Design review of the part built by this model. Coordinates are the model's own, in mm. A direction names the side the tool comes from. Round coordinates to 2 decimals unless told otherwise and drop trailing zeros. Order: outer loops, then holes, each group sorted by start corner. A loop starts at its lowest first (then second) coordinate and runs counter-clockwise, first axis right, second up.
from build123d import *

# Parameters (mm, degrees)
SKETCH_1_W               = 45
SKETCH_1_H               = 80
SKETCH_1_R               = 1.6
EXTRUDE_471_DEPTH        = 20
SKETCH_2_R               = 2.6
CUT_EXTRUDE_665_DEPTH    = 46
SKETCH_3_R               = 5.1
CUT_EXTRUDE_863_DEPTH    = 46
SKETCH_5_W               = 30
SKETCH_5_H               = 20
CUT_EXTRUDE_1108_DEPTH   = 5.5
MIRROR_2_COPY_1_SKETCH_W = 30
MIRROR_2_COPY_1_SKETCH_H = 20
MIRROR_2_COPY_1_DEPTH    = 5.5
FILLET_2_R               = 2
FILLET_5_R               = 5


with BuildPart() as part:
    # 草图1 → Extrude 471 (new body)
    with BuildSketch(Plane(origin=(0, 0, 0), x_dir=(1, 0, 0), z_dir=(0, 1, 0))):
        Rectangle(SKETCH_1_W, SKETCH_1_H)
        with Locations((8, 15)):
            Circle(SKETCH_1_R, mode=Mode.SUBTRACT)
        with Locations((-8, 15)):
            Circle(SKETCH_1_R, mode=Mode.SUBTRACT)
        with Locations((-8, -15)):
            Circle(SKETCH_1_R, mode=Mode.SUBTRACT)
        with Locations((8, -15)):
            Circle(SKETCH_1_R, mode=Mode.SUBTRACT)
    extrude(amount=EXTRUDE_471_DEPTH)

    # 草图2 → Cut-Extrude 665 (cut, through all)
    with BuildSketch(Plane.ZY.offset(22.5)):
        with Locations((0, 10)):
            Circle(SKETCH_2_R)
    extrude(amount=-CUT_EXTRUDE_665_DEPTH, mode=Mode.SUBTRACT)

    # 草图3 → Cut-Extrude 863 (cut, through all)
    with BuildSketch(Plane.ZY.offset(22.5)):
        with Locations((22.5, 10)):
            Circle(SKETCH_3_R)
        with Locations((-22.5, 10)):
            Circle(SKETCH_3_R)
    extrude(amount=-CUT_EXTRUDE_863_DEPTH, mode=Mode.SUBTRACT)

    # 草图5 → Cut-Extrude 1108 (cut)
    with BuildSketch(Plane.ZY.offset(22.5)):
        with Locations((25, 10)):
            Rectangle(SKETCH_5_W, SKETCH_5_H)
    cut_extrude_1108 = extrude(amount=-CUT_EXTRUDE_1108_DEPTH, mode=Mode.SUBTRACT)

    # 镜向1: Cut-Extrude 1108 across plane
    add(cut_extrude_1108.mirror(Plane(origin=(0, 0, 0), x_dir=(0, 0, 1), z_dir=(1, 0, 0))), mode=Mode.SUBTRACT)

    # 镜向2: Cut-Extrude 1108 across plane
    add(cut_extrude_1108.mirror(Plane.XY), mode=Mode.SUBTRACT)

    # 镜向2 copy 1 sketch → 镜向2 copy 1 (cut)
    with BuildSketch(Plane(origin=(22.5, 0, 0), x_dir=(0, 0, -1), z_dir=(1, 0, 0))):
        with Locations((25, 10)):
            Rectangle(MIRROR_2_COPY_1_SKETCH_W, MIRROR_2_COPY_1_SKETCH_H)
    extrude(amount=-MIRROR_2_COPY_1_DEPTH, mode=Mode.SUBTRACT)

    # 圆角2
    fillet_2_edges = [part.edges().sort_by_distance(p)[0] for p in [
        (-22.5, 10, 10),
        (-17, 10, 10),
        (17, 10, 10),
        (22.5, 10, 10),
        (22.5, 10, -10),
        (17, 10, -10),
        (-17, 10, -10),
        (-22.5, 10, -10),
    ]]
    fillet(fillet_2_edges, radius=FILLET_2_R)

    # 圆角5
    fillet_5_edges = [part.edges().sort_by_distance(p)[0] for p in [
        (-17, 10, 40),
        (17, 10, 40),
        (17, 10, -40),
        (-17, 10, -40),
    ]]
    fillet(fillet_5_edges, radius=FILLET_5_R)


solid = part.part
1) Take a section at A-A on z = -22.5. Give the boundary of the cut face in (x, y), plus the area to 3 significant figures.
Results:
outline: (-17, 0) - (17, 0) - (17, 4.9) - (-17, 4.9) - close; (-17, 15.1) - (17, 15.1) - (17, 20) - (-17, 20) - close
area: 333 mm2
2) To check wall thickness, follow line 1 along X through (y, z) = (6, 15); line 2 along Y through (x, z) = (10, -22.5); line 3 along Z through (x, y) = (-2, 7.25). State the ranges of each line that lie inside material, in increasing order.
Results:
line 1: x = -17 to -9.6, -6.4 to 6.4, 9.6 to 17
line 2: y = 0 to 4.9, 15.1 to 20
line 3: z = -40 to -26.8, -18.2 to 18.2, 26.8 to 40
3) The part is to be moulded in two halves that separate along Z. For faces 1 (the face through (15, 10, 39)), 2 (the face through (-9.18, 9.86, 13.92)), 3 (the face through (17, 10, 28)), say which applies: released by +Z, released by -Z, zero draft, split by the parting line, or undercut.
Results:
face 1: released by +Z
face 2: undercut
face 3: zero draft
4) Take a section at C-C on y = 18.25. Give the boundary of the cut face in (x, z).
Results:
outline: (-22.5, -8) arc R2 ccw to (-20.5, -10) - (-19, -10) arc R2 cw to (-17, -12) - (-17, -35) arc R5 ccw to (-12, -40) - (12, -40) arc R5 ccw to (17, -35) - (17, -12) arc R2 cw to (19, -10) - (20.5, -10) arc R2 ccw to (22.5, -8) - (22.5, 8) arc R2 ccw to (20.5, 10) - (19, 10) arc R2 cw to (17, 12) - (17, 35) arc R5 ccw to (12, 40) - (-12, 40) arc R5 ccw to (-17, 35) - (-17, 12) arc R2 cw to (-19, 10) - (-20.5, 10) arc R2 ccw to (-22.5, 8) - close; hole circle Ø3.2 at (-8, -15); hole circle Ø3.2 at (-8, 15); hole circle Ø3.2 at (8, -15); hole circle Ø3.2 at (8, 15)
5) Take a section at B-B on x = -8. Give the boundary of the cut face in (y, z), plus the area to 3 significant figures.
Results:
outline: (0, -40) - (20, -40) - (20, -16.6) - (0, -16.6) - close; (0, -13.4) - (20, -13.4) - (20, 13.4) - (0, 13.4) - close; (0, 16.6) - (20, 16.6) - (20, 40) - (0, 40) - close; hole circle Ø10.2 at (10, -22.5); hole circle Ø10.2 at (10, 22.5); hole circle Ø5.2 at (10, 0)
area: 1,290 mm2
6) Clearance check with flat-ended pins moving along their axes: P1, Ø7, axis at y = 10, z = 0, coming from the -X side; P2, Ø6, axis at y = 11.5, z = -17.5, coming from the -X side; P3, Ø1.2, axis at x = -19.5, y = 8, coming from the +Z side; P4, Ø0.8, axis at x = 19.5, y = 12, coming from the -Z side. State where each tip first meets the part, or that it passes through.
Results:
P1: stops at x = -22.5
P2: stops at x = -17
P3: stops at z = 10
P4: stops at z = -10
7) Take a section at D-D on z = 15. Give the boundary of the cut face in (x, y).
Results:
outline: (-17, 0) - (-9.6, 0) - (-9.6, 20) - (-17, 20) - close; (-6.4, 0) - (6.4, 0) - (6.4, 20) - (-6.4, 20) - close; (9.6, 0) - (17, 0) - (17, 20) - (9.6, 20) - close
8) For faces 4 (the face through (-17, 10, 28)), 5 (the face through (20, 10, 10)), 6 (the face through (6.82, 9.86, 13.92)), list the 3-axis set-ups (+Z, -Z, +X, -X, +Y, -Y) from which the entire face can be reached by the end or side of a thin tool; tool diameter is ignored.
Results:
face 4: +Z, -X, +Y, -Y
face 5: +Z, +X, +Y, -Y
face 6: +Y, -Y
